Build history of the part. All positions in model axes, mm. Face numbers are marked on the shaded views. Give positions to 0.01 mm unless a question says otherwise; leave off trailing zeros. Write each loop counter-clockwise with the first axis right and the second up, starting at its lowest first coordinate (ties: lowest second). Pieces come first, ordered by that corner, then holes.
from build123d import *

# Parameters (mm, degrees)
SKETCH1_W           = 80
SKETCH1_H           = 20
SKETCH1_R           = 2.5
SKETCH1_R_2         = 3
BOSS_EXTRUDE1_DEPTH = 6.35


with BuildPart() as part:
    # Sketch1 → Boss-Extrude1 (new, symmetric)
    with BuildSketch(Plane(origin=(0, 0, 0), x_dir=(1, 0, 0), z_dir=(0, 1, 0))):
        Rectangle(SKETCH1_W, SKETCH1_H)
        with Locations(Location((0, 0, 0), (0, 0, 270))):
            Circle(SKETCH1_R, mode=Mode.SUBTRACT)
        with Locations(Location((-30, 0, 0), (0, 0, 270))):
            Circle(SKETCH1_R_2, mode=Mode.SUBTRACT)
        with Locations(Location((30, 0, 0), (0, 0, 270))):
            Circle(SKETCH1_R_2, mode=Mode.SUBTRACT)
    extrude(amount=BOSS_EXTRUDE1_DEPTH, both=True)


solid = part.part
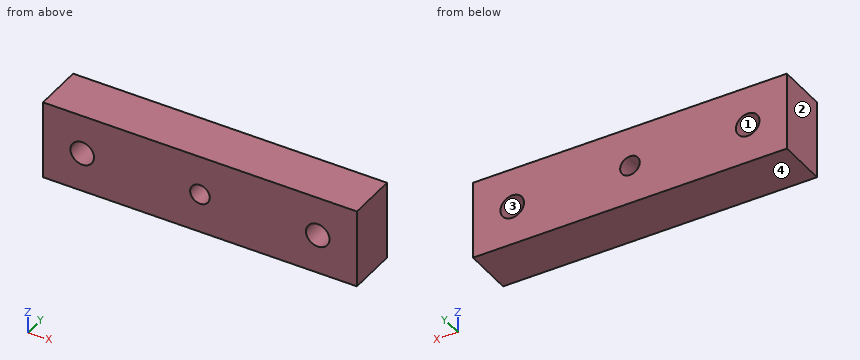
(1) Saw through at A-A, the plane z = 0. List the corners of the cut face in (x, y), plus the area to 3 significant figures.
(2) Saw through at C-C, the plane x = -30. List the corners of the cut face in (y, z).
(3) Saw through at B-B, the plane y = 1. List the corners of the cut face in (x, z), plus the area to 3 significant figures.
(4) Probe line 1 (X direction, y = 4, z = 0); line 2 (X direction, y = 4.25, z = -0.75); line 3 (Z direction, x = 28.5, y = 1.5). List the from-to ranges inside material, lowest first.
(5) Mould opens along Z. For the marked faces 1, 2, 3 and 4 say: +Z half, -Z half, draft (parallel to the pull), parting line (faces both ways), or undercut.
Computed values:
1. outline: (-40, -6.35) - (-33, -6.35) - (-33, 6.35) - (-40, 6.35) - close; (-27, -6.35) - (-2.5, -6.35) - (-2.5, 6.35) - (-27, 6.35) - close; (2.5, -6.35) - (27, -6.35) - (27, 6.35) - (2.5, 6.35) - close; (33, -6.35) - (40, -6.35) - (40, 6.35) - (33, 6.35) - close
1. area: 800 mm2
2. outline: (-6.35, -10) - (6.35, -10) - (6.35, -3) - (-6.35, -3) - close; (-6.35, 3) - (6.35, 3) - (6.35, 10) - (-6.35, 10) - close
3. outline: (-40, -10) - (40, -10) - (40, 10) - (-40, 10) - close; hole circle Ø6 at (-30, 0); hole circle Ø5 at (0, 0); hole circle Ø6 at (30, 0)
3. area: 1,520 mm2
4. line 1: x = -40 to -33, -27 to -2.5, 2.5 to 27, 33 to 40
4. line 2: x = -40 to -32.9, -27.1 to -2.38, 2.38 to 27.1, 32.9 to 40
4. line 3: z = -10 to -2.6, 2.6 to 10
5. face 1: undercut
5. face 2: draft
5. face 3: undercut
5. face 4: -Z half
